Could you check a few things on this model? Use its own coordinates, in mm. Give positions to 0.01 mm unless a question says otherwise; leave off trailing zeros. Put each result on its own line as item: value.
```python
from build123d import *

# Parameters (mm, degrees)
SKETCH1_R           = 38.1
SKETCH1_R_2         = 36.83
SKETCH1_R_3         = 6.35
BOSS_EXTRUDE3_DEPTH = 2.54


with BuildPart() as part:
    # Sketch1 → Boss-Extrude3 (new body)
    # profile 1 of 22: a face of its own
    with BuildSketch(Plane.XY):
        Circle(SKETCH1_R)
        Circle(SKETCH1_R_2, mode=Mode.SUBTRACT)
    # profile 2 of 22: a face of its own
    with BuildSketch(Plane.XY):
        with BuildLine():
            Line((-11.381095903, -35.027411495), (-1.962257914, -6.039208878))
            ThreePointArc((-1.962257914, -6.039208878), (-2.430039796, -5.866635031), (-2.882839673, -5.657891429))
            Line((-2.882839673, -5.657891429), (-16.720470105, -32.815770286))
            ThreePointArc((-16.720470105, -32.815770286), (-14.094230814, -34.026483182), (-11.381095903, -35.027411495))
        make_face()
    # profile 3 of 22: a face of its own
    with BuildSketch(Plane.XY):
        with BuildLine():
            Line((0, -36.83), (0, -6.35))
            ThreePointArc((0, -6.35), (-0.498215258, -6.330425069), (-0.993358853, -6.271820963))
            Line((-0.993358853, -6.271820963), (-5.761481347, -36.376561584))
            ThreePointArc((-5.761481347, -36.376561584), (-2.889648496, -36.716465401), (0, -36.83))
        make_face()
    # profile 4 of 22: a face of its own
    with BuildSketch(Plane.XY):
        with BuildLine():
            ThreePointArc((1.962257914, -6.039208878), (1.48237806, -6.174548995), (0.993358853, -6.271820963))
            Line((0.993358853, -6.271820963), (5.761481347, -36.376561584))
            ThreePointArc((5.761481347, -36.376561584), (8.597792751, -35.812384168), (11.381095903, -35.027411495))
            Line((11.381095903, -35.027411495), (1.962257914, -6.039208878))
        make_face()
    # profile 5 of 22: a face of its own
    with BuildSketch(Plane.XY):
        with BuildLine():
            ThreePointArc((3.732436352, -5.137257914), (3.317865886, -5.414265044), (2.882839673, -5.657891429))
            Line((2.882839673, -5.657891429), (16.720470105, -32.815770286))
            ThreePointArc((16.720470105, -32.815770286), (19.243622138, -31.402737253), (21.648130842, -29.796095903))
            Line((21.648130842, -29.796095903), (3.732436352, -5.137257914))
        make_face()
    # profile 6 of 22: a face of its own
    with BuildSketch(Plane.XY):
        with BuildLine():
            ThreePointArc((5.137257914, -3.732436352), (4.828577882, -4.123995107), (4.490128061, -4.490128061))
            Line((4.490128061, -4.490128061), (26.042742751, -26.042742751))
            ThreePointArc((26.042742751, -26.042742751), (28.005751713, -23.91917162), (29.796095903, -21.648130842))
            Line((29.796095903, -21.648130842), (5.137257914, -3.732436352))
        make_face()
    # profile 7 of 22: a face of its own
    with BuildSketch(Plane.XY):
        with BuildLine():
            ThreePointArc((6.039208878, -1.962257914), (5.866635031, -2.430039796), (5.657891429, -2.882839673))
            Line((5.657891429, -2.882839673), (32.815770286, -16.720470105))
            ThreePointArc((32.815770286, -16.720470105), (34.026483182, -14.094230814), (35.027411495, -11.381095903))
            Line((35.027411495, -11.381095903), (6.039208878, -1.962257914))
        make_face()
    # profile 8 of 22: a face of its own
    with BuildSketch(Plane.XY):
        with BuildLine():
            ThreePointArc((6.35, 0), (6.330425069, -0.498215258), (6.271820963, -0.993358853))
            Line((6.271820963, -0.993358853), (36.376561584, -5.761481347))
            ThreePointArc((36.376561584, -5.761481347), (36.716465401, -2.889648496), (36.83, 0))
            Line((36.83, 0), (6.35, 0))
        make_face()
    # profile 9 of 22: a face of its own
    with BuildSketch(Plane.XY):
        with BuildLine():
            ThreePointArc((6.039208878, 1.962257914), (6.174548995, 1.48237806), (6.271820963, 0.993358853))
            Line((6.271820963, 0.993358853), (36.376561584, 5.761481347))
            ThreePointArc((36.376561584, 5.761481347), (35.812384168, 8.597792751), (35.027411495, 11.381095903))
            Line((35.027411495, 11.381095903), (6.039208878, 1.962257914))
        make_face()
    # profile 10 of 22: a face of its own
    with BuildSketch(Plane.XY):
        with BuildLine():
            Line((-21.648130842, -29.796095903), (-3.732436352, -5.137257914))
            ThreePointArc((-3.732436352, -5.137257914), (-4.123995107, -4.828577882), (-4.490128061, -4.490128061))
            Line((-4.490128061, -4.490128061), (-26.042742751, -26.042742751))
            ThreePointArc((-26.042742751, -26.042742751), (-23.91917162, -28.005751713), (-21.648130842, -29.796095903))
        make_face()
    # profile 11 of 22: a face of its own
    with BuildSketch(Plane.XY):
        with BuildLine():
            Line((-29.796095903, -21.648130842), (-5.137257914, -3.732436352))
            ThreePointArc((-5.137257914, -3.732436352), (-5.414265044, -3.317865886), (-5.657891429, -2.882839673))
            Line((-5.657891429, -2.882839673), (-32.815770286, -16.720470105))
            ThreePointArc((-32.815770286, -16.720470105), (-31.402737253, -19.243622138), (-29.796095903, -21.648130842))
        make_face()
    # profile 12 of 22: a face of its own
    with BuildSketch(Plane.XY):
        with BuildLine():
            Line((-35.027411495, -11.381095903), (-6.039208878, -1.962257914))
            ThreePointArc((-6.039208878, -1.962257914), (-6.174548995, -1.48237806), (-6.271820963, -0.993358853))
            Line((-6.271820963, -0.993358853), (-36.376561584, -5.761481347))
            ThreePointArc((-36.376561584, -5.761481347), (-35.812384168, -8.597792751), (-35.027411495, -11.381095903))
        make_face()
    # profile 13 of 22: a face of its own
    with BuildSketch(Plane.XY):
        with BuildLine():
            Line((-36.83, 0), (-6.35, 0))
            ThreePointArc((-6.35, 0), (-6.330425069, 0.498215258), (-6.271820963, 0.993358853))
            Line((-6.271820963, 0.993358853), (-36.376561584, 5.761481347))
            ThreePointArc((-36.376561584, 5.761481347), (-36.716465401, 2.889648496), (-36.83, 0))
        make_face()
    # profile 14 of 22: a face of its own
    with BuildSketch(Plane.XY):
        with BuildLine():
            Line((-35.027411495, 11.381095903), (-6.039208878, 1.962257914))
            ThreePointArc((-6.039208878, 1.962257914), (-5.866635031, 2.430039796), (-5.657891429, 2.882839673))
            Line((-5.657891429, 2.882839673), (-32.815770286, 16.720470105))
            ThreePointArc((-32.815770286, 16.720470105), (-34.026483182, 14.094230814), (-35.027411495, 11.381095903))
        make_face()
    # profile 15 of 22: a face of its own
    with BuildSketch(Plane.XY):
        with BuildLine():
            Line((-29.796095903, 21.648130842), (-5.137257914, 3.732436352))
            ThreePointArc((-5.137257914, 3.732436352), (-4.828577882, 4.123995107), (-4.490128061, 4.490128061))
            Line((-4.490128061, 4.490128061), (-26.042742751, 26.042742751))
            ThreePointArc((-26.042742751, 26.042742751), (-28.005751713, 23.91917162), (-29.796095903, 21.648130842))
        make_face()
    # profile 16 of 22: a face of its own
    with BuildSketch(Plane.XY):
        with BuildLine():
            Line((-21.648130842, 29.796095903), (-3.732436352, 5.137257914))
            ThreePointArc((-3.732436352, 5.137257914), (-3.317865886, 5.414265044), (-2.882839673, 5.657891429))
            Line((-2.882839673, 5.657891429), (-16.720470105, 32.815770286))
            ThreePointArc((-16.720470105, 32.815770286), (-19.243622138, 31.402737253), (-21.648130842, 29.796095903))
        make_face()
    # profile 17 of 22: a face of its own
    with BuildSketch(Plane.XY):
        with BuildLine():
            Line((-11.381095903, 35.027411495), (-1.962257914, 6.039208878))
            ThreePointArc((-1.962257914, 6.039208878), (-1.48237806, 6.174548995), (-0.993358853, 6.271820963))
            Line((-0.993358853, 6.271820963), (-5.761481347, 36.376561584))
            ThreePointArc((-5.761481347, 36.376561584), (-8.597792751, 35.812384168), (-11.381095903, 35.027411495))
        make_face()
    # profile 18 of 22: a face of its own
    with BuildSketch(Plane.XY):
        with BuildLine():
            ThreePointArc((0, 6.35), (0.498215258, 6.330425069), (0.993358853, 6.271820963))
            Line((0.993358853, 6.271820963), (5.761481347, 36.376561584))
            ThreePointArc((5.761481347, 36.376561584), (2.889648496, 36.716465401), (0, 36.83))
            Line((0, 36.83), (0, 6.35))
        make_face()
    # profile 19 of 22: a face of its own
    with BuildSketch(Plane.XY):
        with BuildLine():
            ThreePointArc((1.962257914, 6.039208878), (2.430039796, 5.866635031), (2.882839673, 5.657891429))
            Line((2.882839673, 5.657891429), (16.720470105, 32.815770286))
            ThreePointArc((16.720470105, 32.815770286), (14.094230814, 34.026483182), (11.381095903, 35.027411495))
            Line((11.381095903, 35.027411495), (1.962257914, 6.039208878))
        make_face()
    # profile 20 of 22: a face of its own
    with BuildSketch(Plane.XY):
        with BuildLine():
            ThreePointArc((3.732436352, 5.137257914), (4.123995107, 4.828577882), (4.490128061, 4.490128061))
            Line((4.490128061, 4.490128061), (26.042742751, 26.042742751))
            ThreePointArc((26.042742751, 26.042742751), (23.91917162, 28.005751713), (21.648130842, 29.796095903))
            Line((21.648130842, 29.796095903), (3.732436352, 5.137257914))
        make_face()
    # profile 21 of 22: a face of its own
    with BuildSketch(Plane.XY):
        with BuildLine():
            ThreePointArc((5.137257914, 3.732436352), (5.414265044, 3.317865886), (5.657891429, 2.882839673))
            Line((5.657891429, 2.882839673), (32.815770286, 16.720470105))
            ThreePointArc((32.815770286, 16.720470105), (31.402737253, 19.243622138), (29.796095903, 21.648130842))
            Line((29.796095903, 21.648130842), (5.137257914, 3.732436352))
        make_face()
    # profile 22 of 22: a face of its own
    with BuildSketch(Plane.XY):
        Circle(SKETCH1_R_3)
    extrude(amount=BOSS_EXTRUDE3_DEPTH)


solid = part.part
```
1. I need wall thicknesses on line 1 (X direction, y = -30, z = 2.1); line 2 (X direction, y = -32.5, z = 0.6); line 3 (X direction, y = 27, z = 2.35). Which ranges of each line are inside material? Lowest first, please.
Recorded:
line 1: x = -23.49 to -21.36, -15.29 to -9.75, -4.75 to 0, 4.75 to 9.75, 15.29 to 23.49
line 2: x = -19.88 to -17.33, -16.56 to -10.56, -5.15 to 0, 5.15 to 10.56, 16.56 to 19.88
line 3: x = -26.88 to -25.05, -19.62 to -13.76, -8.77 to -4.28, 0 to 4.28, 8.77 to 13.76, 19.62 to 26.88
2. I'm going to push flat-ended pins straight in: pin 1 (0.8 mm diameter, centred on y = -24, z = 1, fed in from +X); pin 2 (1 mm diameter, centred on x = 21, y = -13.5, fed in from +Z); pin 3 (1.3 mm diameter, centred on x = 28.5, z = 1.5, fed in from +Y); pin 4 (1 mm diameter, centred on y = 27, z = 0.5, fed in from -X). Where does each tip first touch, or does it pass through?
Recorded:
pin 1: stops at x = 29.91
pin 2: passes through
pin 3: stops at y = 26
pin 4: stops at x = -27.37
3. Thinking about a two-plate mould opening in Y: for faces 1 (the face through (-35.803, 8.637, 1.252)), 2 (the face through (15, 15, 1)), which applies, pulls with the +Y half, pulls with the -Y half, needs draft (parallel to the pull), parting line crosses it, or undercut?
Recorded:
face 1: undercut
face 2: undercut
4. If we section it at A-A (y = 18): Count the separate pieces of the cut face and the enclosed holes in it, then the cut area to 3 significant figures.
Recorded:
separate pieces: 8
enclosed holes: 0
area: 89.0 mm^2
